The listing builds one solid part. Answer for the finished solid, in the listing's coordinates (mm). A direction names the side the tool comes from. Round coordinates to 2 decimals unless told otherwise and drop trailing zeros. Write each loop counter-clockwise with the first axis right and the second up, starting at its lowest first coordinate (ties: lowest second). Pieces come first, ordered by that corner, then holes. Notation, with made-up numbers: M 32,20 L 63,20 A27 cw 63,39 Z; hole C 20.5,-7.75 d1. An arc over 180 degrees is marked long. Write each question's results on one line, items separated by ' | '.
from build123d import *

# Parameters (mm, degrees)
SKETCH_1_R               = 20
EXTRUDE_1_DEPTH          = 5
SKETCH_2_W               = 6.3
SKETCH_2_H               = 6.3
CUT_EXTRUDE_1_DEPTH      = 5
EXTRUDE_START            = 7
SKETCH_4_R               = 20
SKETCH_4_R_2             = 10
EXTRUDE_2_DEPTH          = 7
CUT_EXTRUDE_2_DEPTH      = 20
CUT_EXTRUDE_2_DEPTH_BACK = 20
SKETCH_3_R               = 2.1
SKETCH_5_W               = 3
SKETCH_5_H               = 6
CUT_EXTRUDE_3_DEPTH      = 13
CHAMFER_1_SIZE           = 1
EXTRUDE_START_2          = 20
SKETCH_6_R               = 20
SKETCH_6_R_2             = 18
EXTRUDE_3_DEPTH          = 20
CHAMFER_2_SIZE           = 1
SKETCH_7_R               = 4.25
CUT_EXTRUDE_4_DEPTH      = 2
SKETCH_8_W               = 14
SKETCH_8_H               = 14
EXTRUDE_4_DEPTH          = 5.5
SKETCH_9_W               = 6.3
SKETCH_9_H               = 6.3
CUT_EXTRUDE_5_DEPTH      = 10
CUT_EXTRUDE_6_DEPTH      = 6
CUT_EXTRUDE_6_DEPTH_BACK = 5
SKETCH_10_W              = 3
SKETCH_10_H              = 5
FILLET_1_R               = 4
FILLET_2_R               = 2
SKETCH_11_W              = 12.7
SKETCH_11_H              = 12.7
SKETCH_11_W_2            = 6.3
SKETCH_11_H_2            = 6.3
EXTRUDE_5_DEPTH          = 20
CHAMFER_3_SIZE           = 2.5
SKETCH_12_R              = 1.65
CUT_EXTRUDE_7_DEPTH      = 20
FILLET_3_R               = 2.5


with BuildPart() as part:
    # 草图1 → 凸台-拉伸1 (new body)
    with BuildSketch(Plane(origin=(0, 0, 0), x_dir=(0, 0, -1), z_dir=(1, 0, 0))):
        Circle(SKETCH_1_R)
    extrude(amount=EXTRUDE_1_DEPTH)

    # 草图2 → 切除-拉伸1 (cut)
    with BuildSketch(Plane(origin=(5, 0, 0), x_dir=(0, 0, -1), z_dir=(1, 0, 0))):
        Rectangle(SKETCH_2_W, SKETCH_2_H)
    extrude(amount=-CUT_EXTRUDE_1_DEPTH, mode=Mode.SUBTRACT)

    # 草图4 → 凸台-拉伸2 (add)
    with BuildSketch(Plane.ZY.offset(EXTRUDE_START)):
        Circle(SKETCH_4_R)
        Circle(SKETCH_4_R_2, mode=Mode.SUBTRACT)
    extrude(amount=-EXTRUDE_2_DEPTH)

    # 草图3 → 切除-拉伸2 (cut, two sides: drawn at the far end of the back side and taken through both)
    with BuildSketch(Plane.ZY.offset(-CUT_EXTRUDE_2_DEPTH_BACK)):
        with Locations(Location((9.899494937, -9.899494937, 0), (0, 0, 180))):
            Circle(SKETCH_3_R)
        with Locations(Location((-9.899494937, -9.899494937, 0), (0, 0, 180))):
            Circle(SKETCH_3_R)
        with Locations(Location((-9.899494937, 9.899494937, 0), (0, 0, 180))):
            Circle(SKETCH_3_R)
        with Locations(Location((9.899494937, 9.899494937, 0), (0, 0, 180))):
            Circle(SKETCH_3_R)
    extrude(amount=CUT_EXTRUDE_2_DEPTH + CUT_EXTRUDE_2_DEPTH_BACK, mode=Mode.SUBTRACT)

    # 草图5 → 切除-拉伸3 (cut)
    with BuildSketch(Plane(origin=(5, 0, 0), x_dir=(0, 0, -1), z_dir=(1, 0, 0))):
        with Locations((14, 0)):
            Rectangle(SKETCH_5_W, SKETCH_5_H)
    extrude(amount=-CUT_EXTRUDE_3_DEPTH, mode=Mode.SUBTRACT)

    # 倒角1
    chamfer_1_edges = [part.edges().sort_by_distance(p)[0] for p in [
        (-7, -3, -14),
        (-7, 0, -15.5),
        (-7, 3, -14),
        (-7, 0, -12.5),
    ]]
    chamfer(chamfer_1_edges, length=CHAMFER_1_SIZE)

    # 草图6 → 凸台-拉伸3 (add)
    with BuildSketch(Plane.ZY.offset(7).offset(EXTRUDE_START_2)):
        Circle(SKETCH_6_R)
        Circle(SKETCH_6_R_2, mode=Mode.SUBTRACT)
    extrude(amount=-EXTRUDE_3_DEPTH)

    # 倒角2
    chamfer_2_edges = [part.edges().sort_by_distance(p)[0] for p in [
        (-27, 0, -18),
    ]]
    chamfer(chamfer_2_edges, length=CHAMFER_2_SIZE)

    # 草图7 → 切除-拉伸4 (cut)
    with BuildSketch(Plane(origin=(5, 0, 0), x_dir=(0, 0, -1), z_dir=(1, 0, 0))):
        with Locations((-9.899494937, 9.899494937)):
            Circle(SKETCH_7_R)
        with Locations((9.899494937, 9.899494937)):
            Circle(SKETCH_7_R)
        with Locations((9.899494937, -9.899494937)):
            Circle(SKETCH_7_R)
        with Locations((-9.899494937, -9.899494937)):
            Circle(SKETCH_7_R)
    extrude(amount=-CUT_EXTRUDE_4_DEPTH, mode=Mode.SUBTRACT)

    # 草图8 → 凸台-拉伸4 (add)
    with BuildSketch(Plane(origin=(5, 0, 0), x_dir=(0, 0, -1), z_dir=(1, 0, 0))):
        Rectangle(SKETCH_8_W, SKETCH_8_H)
    extrude(amount=EXTRUDE_4_DEPTH)

    # 草图9 → 切除-拉伸5 (cut)
    with BuildSketch(Plane.ZY.offset(-5)):
        Rectangle(SKETCH_9_W, SKETCH_9_H)
    extrude(amount=-CUT_EXTRUDE_5_DEPTH, mode=Mode.SUBTRACT)

    # 草图10 → 切除-拉伸6 (cut, two sides: drawn at the far end of the back side and taken through both)
    with BuildSketch(Plane(origin=(0, 0, -7), x_dir=(-1, 0, 0), z_dir=(0, 0, -1)).offset(-CUT_EXTRUDE_6_DEPTH_BACK)):
        with Locations((-5, 0)):
            Rectangle(SKETCH_10_W, SKETCH_10_H)
    extrude(amount=CUT_EXTRUDE_6_DEPTH + CUT_EXTRUDE_6_DEPTH_BACK, mode=Mode.SUBTRACT)

    # 圆角1
    fillet_1_edges = [part.edges().sort_by_distance(p)[0] for p in [
        (3.5, 0, -12.5),
    ]]
    fillet(fillet_1_edges, radius=FILLET_1_R)

    # 圆角2
    fillet_2_edges = [part.edges().sort_by_distance(p)[0] for p in [
        (6.5, 0, -3.15),
    ]]
    fillet(fillet_2_edges, radius=FILLET_2_R)

    # 草图11 → 凸台-拉伸5 (add)
    with BuildSketch(Plane(origin=(10.5, 0, 0), x_dir=(0, 0, -1), z_dir=(1, 0, 0))):
        Rectangle(SKETCH_11_W, SKETCH_11_H)
        Rectangle(SKETCH_11_W_2, SKETCH_11_H_2, mode=Mode.SUBTRACT)
    extrude(amount=EXTRUDE_5_DEPTH)

    # 倒角3
    chamfer_3_edges = [part.edges().sort_by_distance(p)[0] for p in [
        (30.5, 0, 6.35),
        (30.5, -6.35, 0),
        (30.5, 0, -6.35),
        (30.5, 6.35, 0),
    ]]
    chamfer(chamfer_3_edges, length=CHAMFER_3_SIZE)

    # 草图12 → 切除-拉伸7 (cut)
    with BuildSketch(Plane.XZ.offset(6.35)):
        with Locations(Location((20.5, 0, 0), (0, 0, 270))):
            Circle(SKETCH_12_R)
    extrude(amount=-CUT_EXTRUDE_7_DEPTH, mode=Mode.SUBTRACT)

    # 圆角3
    fillet_3_edges = [part.edges().sort_by_distance(p)[0] for p in [
        (19.25, 6.35, 6.35),
        (19.25, 6.35, -6.35),
        (19.25, -6.35, -6.35),
        (19.25, -6.35, 6.35),
    ]]
    fillet(fillet_3_edges, radius=FILLET_3_R)


solid = part.part
1) Section B-B (x = -4) is taken. Determine the outline of the cut face in (y, z).
Return value:
outline: C 0,0 d40; hole C -9.9,-9.9 d4.2; hole C -9.9,9.9 d4.2; hole C 0,0 d20; hole M -3,-15.5 L 3,-15.5 L 3,-12.5 L -3,-12.5 Z; hole C 9.9,-9.9 d4.2; hole C 9.9,9.9 d4.2
2) Each of these flat-tipped pins is pushed along its axis until it touches: pin 1 (6 mm diameter, centred on y = -2, z = 3, fed in from +X); pin 2 (6 mm diameter, centred on x = -16.5, y = -12, fed in from +Z); pin 3 (10 mm diameter, centred on y = -9.9, z = 9.9, fed in from +X); pin 4 (2.5 mm diameter, centred on y = -10.5, z = -8.5, fed in from +X). Where does it stop, or does it pass through?
Return value:
pin 1: x = 30.5 | pin 2: z = 17.86 | pin 3: x = 10.5 | pin 4: x = 3
3) Section D-D (x = 9.5) is taken. Determine the outline of the cut face in (y, z).
Return value:
outline: M -7,-7 L 7,-7 L 7,7 L -7,7 Z; hole M -3.15,-3.15 L 3.15,-3.15 L 3.15,3.15 L -3.15,3.15 Z
4) The mould has two halves that part along X. Classify faces 1 (the face through (5, -9, 0)), 2 (the face through (4, -2.5, -7)), 3 (the face through (-3.55, -9.76, -2.17)): +X half, -X half, draft (parallel to the pull), parting line (faces both ways), or undercut.
Return value:
face 1: +X half | face 2: undercut | face 3: draft
5) Section C-C (y = 0) is taken. State how many separate pieces and enclosed holes the cut face has, then the cut area to 3 significant figures.
Return value:
separate pieces: 4 | enclosed holes: 0 | area: 491 mm²
6) A tool of negligible diameter and unlimited length cuts with its end or side. For faces 4 (the face through (19.744, -5.637, -5.598)), 5 (the face through (7.07, 0.04, -3.75)), 6 (the face through (8, 0, -7)), from which of +Z, -Z, +X, -X, +Y, -Y can it reach the whole face along a straight path? Write none if from no direction.
Return value:
face 4: -Z, +X, -Y | face 5: none | face 6: -Z, +X, +Y, -Y
7) Find the intervals of material crossed by line 1 (Y direction, x = 4, z = 12); line 2 (Y direction, x = -3.5, z = -11); line 3 (X direction, y = -4, z = 11), in increasing order.
Return value:
line 1: -16 to -13.59, -6.2 to 6.2, 13.59 to 16 | line 2: -16.7 to -11.69, -8.11 to 8.11, 11.69 to 16.7 | line 3: -7 to 5
8) Section A-A (x = 20.5) is taken. Determine the outline of the cut face in (y, z).
Return value:
outline: M -6.35,-3.85 A2.5 ccw -3.85,-6.35 L 3.85,-6.35 A2.5 ccw 6.35,-3.85 L 6.35,-1.65 L 3.15,-1.65 L 3.15,-3.15 L -3.15,-3.15 L -3.15,-1.65 L -6.35,-1.65 Z; M -6.35,1.65 L -3.15,1.65 L -3.15,3.15 L 3.15,3.15 L 3.15,1.65 L 6.35,1.65 L 6.35,3.85 A2.5 ccw 3.85,6.35 L -3.85,6.35 A2.5 ccw -6.35,3.85 Z
